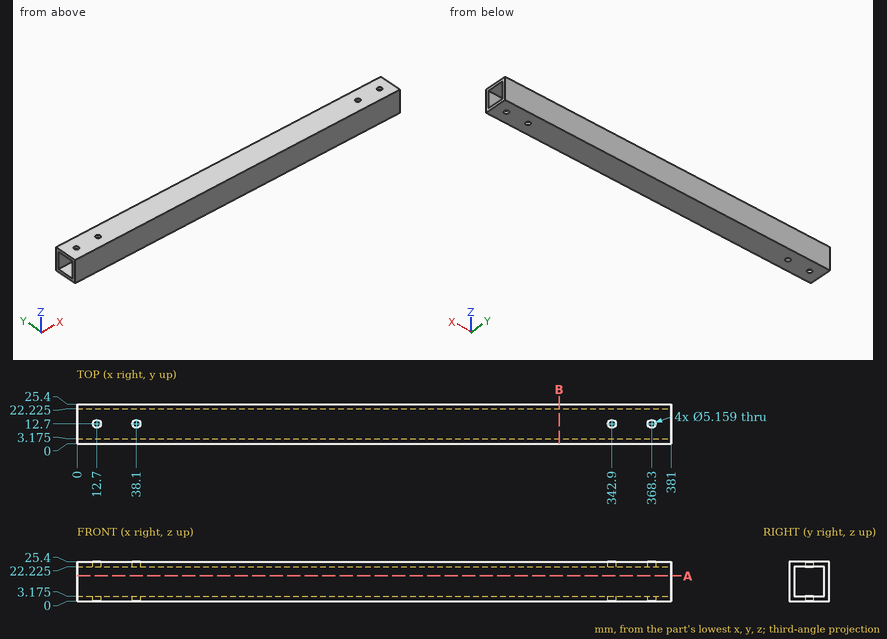
Can you work these out from the drawing? Everything is in mm from the part's minimum corner. Give positions to 0.01 mm unless a question says otherwise; leave off trailing zeros. Loops run counter-clockwise (first coordinate to the right, second up) from the corner with the lowest first, then second, coordinate; pieces in that order, holes last. Notation, with made-up numbers: (71.5, 79) - (105.5, 79) arc R14 ccw to (105.5, 103) - close; hole circle Ø6 at (36, 47). An arc over 180 degrees is marked (long way). Answer as a JSON object with one key per item and string values.
Q1. If I drill on L1, parallel to Z at x = 18, y = 19.75 (1 decimal); L2, parallel to Y at x = 12.7, z = 1.05, over which ranges is the centre line in solid material (lowest first)?
Geometry says:
{"L1": "0 to 3.2, 22.2 to 25.4", "L2": "0 to 10.12, 15.28 to 25.4"}
Q2. Imagine slicing it at A-A on z = 16.25. Write out the boundary of the cut face in (x, y) (1 decimal).
Geometry says:
{"outline": "(0, 0) - (381, 0) - (381, 3.2) - (0, 3.2) - close; (0, 22.2) - (381, 22.2) - (381, 25.4) - (0, 25.4) - close"}
Q3. Imagine slicing it at B-B on x = 309. Write out the boundary of the cut face in (y, z) (1 decimal), plus the area to 3 significant figures.
Geometry says:
{"outline": "(0, 0) - (25.4, 0) - (25.4, 25.4) - (0, 25.4) - close; hole (3.2, 3.2) - (22.2, 3.2) - (22.2, 22.2) - (3.2, 22.2) - close", "area": "282 mm²"}
